Input: part model. Units: mm. Frame: model coordinates. A direction names the side the tool comes from. Round coordinates to 2 decimals unless told otherwise and drop trailing zeros. Write each loop counter-clockwise with the first axis right and the second up, starting at its lowest first coordinate (ties: lowest second). Pieces come first, ordered by that corner, then holes. Notation, with made-up numbers: (5, -35.75) -> (35, -35.75) arc R16 ccw to (35, -31.75) -> close; hole circle Ø11 at (-10, 82.5). An arc over 180 degrees is marked (long way). Write item = value, one per line. Start each with the question number.
```python
from build123d import *

# Parameters (mm, degrees)
SKETCH1_R                = 4
BOSS_EXTRUDE1_DEPTH      = 6
BOSS_EXTRUDE1_DEPTH_BACK = 6
SKETCH2_W                = 1.5
SKETCH2_H                = 4.5
CUT_EXTRUDE1_DEPTH       = 24


with BuildPart() as part:
    # Sketch1 → Boss-Extrude1 (new body, two sides)
    with BuildSketch(Plane(origin=(0, 0, 0), x_dir=(1, 0, 0), z_dir=(0, 1, 0))) as boss_extrude1_sk:
        with BuildLine():
            Line((-4, 3), (-7.5, 3))
            Line((-7.5, 3), (-7.5, -3))
            Line((-7.5, -3), (-4, -3))
            ThreePointArc((-4, -3), (-3.548890872, -3.522126287), (-3.030194493, -3.977175044))
            Line((-3.030194493, -3.977175044), (18, -20))
            Line((18, -20), (20, -20))
            Line((20, -20), (20, -1.905552368))
            Line((20, -1.905552368), (20, 20))
            Line((20, 20), (18, 20))
            Line((18, 20), (-3.030194493, 3.977175044))
            ThreePointArc((-3.030194493, 3.977175044), (-3.548890872, 3.522126287), (-4, 3))
        make_face()
        Circle(SKETCH1_R, mode=Mode.SUBTRACT)
        with BuildLine():
            Line((4.898979486, 1), (18, 1))
            Line((18, 1), (18, 18.114239399))
            Line((18, 18.114239399), (0.719134947, 4.948014241))
            ThreePointArc((0.719134947, 4.948014241), (3.433293835, 3.634899372), (4.898979486, 1))
        make_face(mode=Mode.SUBTRACT)
        with BuildLine():
            Line((4.898979486, -1), (18, -1))
            Line((18, -1), (18, -18.114239399))
            Line((18, -18.114239399), (0.719134947, -4.948014241))
            ThreePointArc((0.719134947, -4.948014241), (3.433293835, -3.634899372), (4.898979486, -1))
        make_face(mode=Mode.SUBTRACT)
    extrude(amount=BOSS_EXTRUDE1_DEPTH)
    extrude(boss_extrude1_sk.sketch, amount=-BOSS_EXTRUDE1_DEPTH_BACK)

    # Sketch2 → Cut-Extrude1 (cut, through all)
    with BuildSketch(Plane(origin=(0, 0, -3), x_dir=(-1, 0, 0), z_dir=(0, 0, -1))):
        with Locations((5.15, 0)):
            Rectangle(SKETCH2_W, SKETCH2_H)
    extrude(amount=-CUT_EXTRUDE1_DEPTH, mode=Mode.SUBTRACT)


solid = part.part
```
1. Section D-D (x = 9.25). Output: boundary loops of the cut face in (y, z).
2. Section A-A (z = 0). Output: boundary loops of the cut face in (x, y), then the cut area to 3 significant figures.
3. Section B-B (x = 0.25). Output: boundary loops of the cut face in (y, z), then the cut area to 3 significant figures.
4. Line query: line 1 along X through (y, z) = (3.45, 0); line 2 along X through (y, z) = (-0.5, -1.5); line 3 along Z through (x, y) = (8, 4.75). Output: solid intervals per line, ascending.
5. Mould query, pull axis Z, two halves, no side actions, for faces 1 (the flat face through (7.63, 0.08, -12.1)), 2 (the cylindrical face through (3, 0, 4)), 3 (the flat face through (-6.2, 0.1, 3)). Classes: pulls with the +Z half, pulls with the -Z half, needs draft (parallel to the pull), parting line crosses it, or undercut.
6. Pin query (flat end, axial travel): P1, Ø4, axis at y = -3, z = 7, coming from the -X side; P2, Ø6.5, axis at y = 4, z = -6.5, coming from the -X side; P3, Ø1, axis at x = 9.5, y = -1.5, coming from the +Z side; P4, Ø9, axis at x = 0, z = 0, coming from the +Y side. Return the tip coordinate at first contact, or that it passes through.
7. Reachability of faces 4 (the flat face through (-5.9, 0, 0)), 5 (the flat face through (11, 0, 1)), 6 (the flat face through (19, 0, -20)), 7 (the flat face through (-6.1, 0.1, -3)) from +Z, -Z, +X, -X, +Y, -Y: full face, straight path, thin tool, end or side. Return the list, or none.
8. Section C-C (y = -4.5). Output: boundary loops of the cut face in (x, z).
Check sheet entries:
q1.outline = (-6, -13.33) -> (6, -13.33) -> (6, -11.45) -> (-6, -11.45) -> close; (-6, -1) -> (6, -1) -> (6, 1) -> (-6, 1) -> close; (-6, 11.45) -> (6, 11.45) -> (6, 13.33) -> (-6, 13.33) -> close
q2.outline = (-7.5, -6) -> (-4, -6) -> (-4, 6) -> (-7.5, 6) -> close; (4, -6) -> (20, -6) -> (20, 6) -> (4, 6) -> close; hole (-5.9, -2.25) -> (-4.4, -2.25) -> (-4.4, 2.25) -> (-5.9, 2.25) -> close
q2.area = 227 mm2
q3.outline = (-6, -6.48) -> (6, -6.48) -> (6, -3.99) -> (-6, -3.99) -> close; (-6, 3.99) -> (6, 3.99) -> (6, 6.48) -> (-6, 6.48) -> close
q3.area = 59.6 mm2
q4.line_1 = -7.5 to -4, 4 to 20
q4.line_2 = -7.5 to -5.9, -4.4 to -3.71, 3.71 to 4.77, 18 to 20
q4.line_3 = -12.38 to -10.5, -1 to 1, 10.5 to 12.38
q5.face_1 = pulls with the -Z half
q5.face_2 = undercut
q5.face_3 = pulls with the +Z half
q6.P1 = -1.69
q6.P2 = -3.8
q6.P3 = 13.9
q6.P4 = 6
q7.face_4 = +Z, -Z
q7.face_5 = +Y, -Y
q7.face_6 = -Z, +X, -X, +Y, -Y
q7.face_7 = -Z, -X, +Y, -Y
q8.outline = (-7.5, -3) -> (-4, -3) arc R5 ccw to (-3.03, -3.98) -> (18, -20) -> (20, -20) -> (20, 20) -> (18, 20) -> (-3.03, 3.98) arc R5 ccw to (-4, 3) -> (-7.5, 3) -> close; hole circle Ø8 at (0, 0); hole (0.72, -4.95) -> (18, -18.11) -> (18, -1) -> (4.9, -1) arc R5 cw to start; hole (0.72, 4.95) arc R5 cw to (4.9, 1) -> (18, 1) -> (18, 18.11) -> close
